Autodesk Fusion 360 part; units mm, degrees
sketch "Sketch1" plane through (0, 0, 0) normal (0, 0, 1) x (1, 0, 0)
  circle A0 centre (0, 0) radius 7
  circle A1 centre (0, 0) radius 10
  dimension "d1" = 3
  dimension "d2" = 14
extrude "Extrude1" add sketch "Sketch1" along normal blind 10
extrude "Extrude2" add sketch "Sketch1" against normal blind 2 contours A0 | A1
fillet "Fillet1" radius 3 1 edges at (-9.3233, 3.6162, -2)
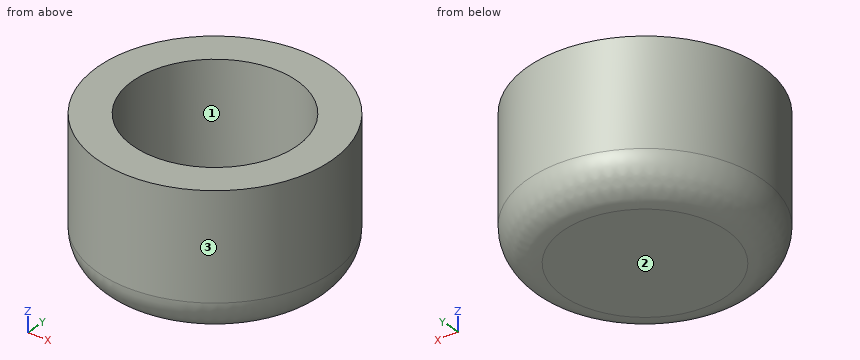
The listing builds one solid part. Answer for the finished solid, in the listing's coordinates (mm). Face numbers are marked on the shaded views. Give positions to 0.01 mm unless a question says otherwise; leave off trailing zeros. Order: outer loops, then holes, each group sorted by start corner. A loop starts at its lowest first (then second) coordinate and runs counter-clockwise, first axis right, second up. Notation, with made-up numbers: (29, 39.25) -> (64, 39.25) arc R34 ccw to (64, 76.25) -> close; hole circle Ø11 at (46.25, 49). An arc over 180 degrees is marked (long way). Answer as a JSON object with one key per item and string values. Group by question number.
Item 1: Determine the mould class of the marked faces 1, 2 and 3 for opening direction Y: pulls with the +Y half, pulls with the -Y half, needs draft (parallel to the pull), parting line crosses it, or undercut.
Item 2: The part is cut by section A-A on z = 6. Write down the section's boundary in (x, y), and give its area (3 significant figures).
Item 3: Flat-ended cylindrical pins translate along their axes: pin 1 (6 mm diameter, centred on x = -4.5, z = 8, fed in from +Y); pin 2 (4 mm diameter, centred on y = 3, z = 3, fed in from +X); pin 3 (2 mm diameter, centred on x = -5, z = 3, fed in from -Y). Find the tip coordinate at first contact, or state that the pin passes through.
Item 4: Consider L1, parallel to Y at x = 0, z = 4.25; L2, parallel to Z at x = 0.5, y = -5.5; L3, parallel to Y at x = 5.75, z = 7. Determine where each line is inside the solid, lowest interval first. Write a range as from..to.
Result set:
{
 "1": {"face 1": "undercut", "face 2": "needs draft", "face 3": "parting line crosses it"},
 "2": {"outline": "circle Ø20 at (0, 0); hole circle Ø14 at (0, 0)", "area": "160 mm²"},
 "3": {"pin 1": "y = 9.89", "pin 2": "x = 9.95", "pin 3": "y = -9.17"},
 "4": {"L1": "-10..-7, 7..10", "L2": "-2..0", "L3": "-8.18..-3.99, 3.99..8.18"}
}
